Verification items for the finished model (mm, model axes). Coordinates: 2 decimals unless noted, no trailing zeros. Loops run counter-clockwise (first coordinate to the right, second up) from the corner with the lowest first, then second, coordinate; pieces in that order, holes last.
Q1. Sectioned sample at B-B (y = 2.5). Count the separate pieces of the cut face and the enclosed holes in it, then the cut area to 3 significant figures.
Q2. Material ranges on probe 1 along Z at (x, y) = (20.5, 1.7); probe 2 along X at (y, z) = (2.15, 69); probe 3 along X at (y, z) = (0.4, 172.5), recorded low to high.
Q3. Go/stop test with flat-tipped pins: P1, Ø0.9, axis at x = 152.5, y = 1.5, coming from the -Z side; P2, Ø1.5, axis at y = 2, z = 140.5, coming from the -X side; P3, Ø1.5, axis at x = -47.5, y = 1, coming from the -Z side. Record where each tip stops, or that it passes through.
Q4. Sectioned sample at A-A (z = 71.5). Enter the section's corners in (x, y).
Q5. Sectioned sample at C-C (x = -31.5). Enter the section's corners in (y, z).
Autodesk Inventor part; units mm, degrees
ref_plane "YZ Plane" through (0, 0, 0) normal (1, 0, 0) x (0, 1, 0)
ref_plane "XZ Plane" through (0, 0, 0) normal (0, 1, 0) x (-1, 0, 0)
ref_plane "XY Plane" through (0, 0, 0) normal (0, 0, 1) x (1, 0, 0)
sketch "Sketch1" plane through (0, 0, 0) normal (0, 1, 0) x (-1, 0, 0)
  line L0 (16.7044, 65.1664) -> (16.7044, 62.1664)
  line L1 (-20.3174, 65.1664) -> (-20.3174, 62.1664)
  line L2 (-51.677, 65.1664) -> (-51.677, 62.1664)
  line L3 (-144.9395, 65.1664) -> (-144.9395, 62.1664)
  line L4 (-107.9177, 65.1664) -> (-107.9177, 62.1664)
  line L5 (-76.5581, 65.1664) -> (-76.5581, 62.1664)
  line L6 (45.8824, 65.1664) -> (16.7044, 65.1664)
  line L7 (-64.1176, 62.1664) -> (-51.677, 62.1664)
  line L8 (-20.3174, 62.1664) -> (16.7044, 62.1664)
  line L9 (16.7044, 62.1664) -> (-20.3174, 62.1664)
  line L10 (-20.3174, 65.1664) -> (-51.677, 65.1664)
  line L11 (-51.677, 62.1664) -> (-76.5581, 62.1664)
  line L12 (-107.9177, 62.1664) -> (-144.9395, 62.1664)
  line L13 (-64.1176, 62.1664) -> (-76.5581, 62.1664)
  line L14 (-76.5581, 65.1664) -> (-107.9177, 65.1664)
  line L15 (-144.9395, 65.1664) -> (-174.1176, 65.1664)
  line L16 (48.8824, 80.1664) -> (48.8824, 95.1664)
  line L17 (48.8824, 95.1664) -> (45.8824, 95.1664)
  line L18 (48.8824, 80.1664) -> (45.8824, 80.1664)
  line L19 (48.8824, 115.1664) -> (45.8824, 115.1664)
  line L20 (48.8824, 130.1664) -> (45.8824, 130.1664)
  line L21 (-177.1176, 130.1664) -> (-174.1176, 130.1664)
  line L22 (-177.1176, 115.1664) -> (-174.1176, 115.1664)
  line L23 (-177.1176, 95.1664) -> (-174.1176, 95.1664)
  line L24 (-177.1176, 80.1664) -> (-174.1176, 80.1664)
  line L25 (45.8824, 80.1664) -> (45.8824, 65.1664)
  line L26 (48.8824, 115.1664) -> (48.8824, 130.1664)
  line L27 (45.8824, 145.1664) -> (45.8824, 130.1664)
  line L28 (45.8824, 115.1664) -> (45.8824, 95.1664)
  line L29 (-174.1176, 65.1664) -> (-174.1176, 80.1664)
  line L30 (-174.1176, 95.1664) -> (-174.1176, 115.1664)
  line L31 (-174.1176, 130.1664) -> (-174.1176, 145.1664)
  line L32 (-177.1176, 80.1664) -> (-177.1176, 95.1664)
  line L33 (-177.1176, 115.1664) -> (-177.1176, 130.1664)
  line L34 (-213.0378, 187.8664) -> (84.2595, 187.8664)
  line L35 (-177.1176, 187.8664) -> (-177.1176, 145.1664)
  line L36 (-177.1176, 145.1664) -> (-174.1176, 145.1664)
  line L37 (48.8824, 187.8664) -> (48.8824, 145.1664)
  line L38 (48.8824, 145.1664) -> (45.8824, 145.1664)
  circle A0 centre (-81.336, 175.651) radius 2.5
  circle A1 centre (-90.2887, 130.1664) radius 2.5
  circle A2 centre (-64.1176, 173.151) radius 2.5
  circle A3 centre (-46.8991, 175.651) radius 2.5
  circle A4 centre (-37.9465, 130.1664) radius 2.5
  point P0 (0, 0)
  point P1 (48.8824, 62.1664)
  point P2 (-126.4286, 62.1664)
  point P3 (-161.0285, 65.1664)
  point P4 (-177.1176, 122.6664)
  point P5 (48.8824, 122.6664)
  point P6 (-76.5581, 63.6664)
  point P7 (-51.677, 63.6664)
  dimension "d1" = 15
  dimension "d3" = 220
  dimension "d4" = 226
  dimension "d5" = 20
  dimension "d6" = 15
  dimension "d7" = 15
  dimension "d9" = 15
  dimension "d10" = 29.178
  dimension "d11" = 37.0218
  dimension "d12" = 31.3596
  dimension "d13" = 24.8811
  dimension "d14" = 31.3596
  dimension "d16" = 37.0218
  dimension "d17" = 29.178
  dimension "d18" = 15
  dimension "d19" = 15
  dimension "d20" = 20
  dimension "d21" = 15
  dimension "d22" = 15
  dimension "d23" = 3
  dimension "d24" = 3
  dimension "d27" = 122.7
  dimension "d28" = 5
  dimension "d29" = 5
  dimension "d30" = 65
  dimension "d31" = 5
extrude "Extrusion1" add sketch "Sketch1" along normal blind 3
properties part number "mieng_mat_3mm"
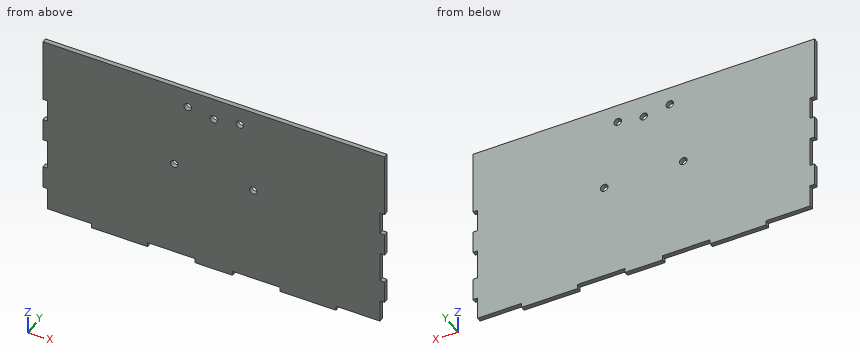
Geometry check:
1. separate pieces: 1
1. enclosed holes: 5
1. area: 27,600 mm2
2. probe 1: z = 65.17 to 187.87
2. probe 2: x = -45.88 to 174.12
2. probe 3: x = -48.88 to 61.7, 66.53 to 177.12
3. P1: stops at z = 65.17
3. P2: stops at x = -45.88
3. P3: stops at z = 80.17
4. outline: (-45.88, 0) - (174.12, 0) - (174.12, 3) - (-45.88, 3) - close
5. outline: (0, 65.17) - (3, 65.17) - (3, 187.87) - (0, 187.87) - close
